Source: CAD feature listing. Evaluate the final solid. Frame: model axes, mm. Face numbers are marked on the shaded views. A direction names the side the tool comes from. Round coordinates to 2 decimals unless told otherwise and drop trailing zeros. Order: outer loops, then holes, each group sorted by start corner. A loop starts at its lowest first (then second) coordinate and runs counter-clockwise, first axis right, second up. Notation, with made-up numbers: (56, 32.25) - (100, 32.25) arc R12 ccw to (100, 37.25) - close; hole circle Ø11 at (60, -22.75). An arc over 180 degrees is marked (long way). Use one line per item in the form item = value. Start each with the question number.
Q1. Cut plane B-B, the plane y = 32. Return the cut outline in (x, z).
Q2. Ray query, line 1 (X direction, y = 16, z = 96.5); line 2 (Y direction, x = -37, z = 23); line 3 (Z direction, x = -62, y = 70). Return the intervals inside material, ascending. Write a range as [from, to].
Q3. Set-up query: the marked faces 1 and 2. Return all of +Z, -Z, +X, -X, +Y, -Y with unobstructed straight access to the full face (end or side cutting, diameter ignored); none if empty.
Q4. Cut plane C-C, the plane z = 8.5. Return the cut outline in (x, y), and give its area (3 significant figures).
Q5. Cut plane D-D, the plane x = -61.5. Return the cut outline in (y, z).
Q6. Draft query along Y for the marked faces 3, 4 and 5. Return one class per face: released by +Y, released by -Y, zero draft, split by the parting line, or undercut.
Q7. Cut plane A-A, the plane x = -28.5. Return the cut outline in (y, z), and give its area (3 significant figures).
Q8. Pin query (flat end, axial travel): pin 1 Ø0.8 at (y, z) = (0.5, 63.5) entering from -X; pin 2 Ø3 at (x, z) = (-52, 51.5) entering from -Y; pin 3 Ø1.5 at (x, y) = (-27.5, 50) entering from +Z. Return the tip coordinate at first contact, or that it passes through.
from build123d import *

# Parameters (mm, degrees)
F0_W     = 83.5
F0_H     = 82.5
F1_DEPTH = 116
F3_DEPTH = 25
F4_R     = 3
F5_DEPTH = 2
F6_R     = 4.99999


# Not quite as in the source:
# - a fillet or chamfer is up to 0.001 mm smaller than in the source, because OpenCascade refuses the exact size


with BuildPart() as f1:
    # F0 (on Top) → F1 (new body)
    with BuildSketch(Plane.XY):
        with Locations((-41.75, 41.25)):
            Rectangle(F0_W, F0_H)
        Polygon((-2, 1.5), (-43.8047535717, 1.5), (-81.5, 1.5), (-81.5, 41.25), (-81.5, 80.5), (-41.75, 80.5), (-2, 80.5), (-2, 41.25), align=None, mode=Mode.SUBTRACT)
    extrude(amount=F1_DEPTH)

    # F2 (on Front) → F3 (cut)
    with BuildSketch(Plane.XZ):
        Polygon((-5, 111), (-78.5, 111), (-78.5, 20), (-41.75, 20), (-34.1152064502, 32.9003408551), (-5, 32.9003408551), align=None)
    extrude(amount=-F3_DEPTH, mode=Mode.SUBTRACT)

    # F4
    f4_edges = [f1.edges().sort_by_distance(p)[0] for p in [
        (-34.115206, 0.75, 32.900341),
    ]]
    fillet(f4_edges, radius=F4_R)

    # F0 (on Top) → F5 (join)
    with BuildSketch(Plane.XY):
        Polygon((-81.5, 1.5), (-43.8047535717, 1.5), (-2, 1.5), (-2, 41.25), (-2, 80.5), (-41.75, 80.5), (-81.5, 80.5), (-81.5, 41.25), align=None)
    extrude(amount=F5_DEPTH)

    # F6 (radius 5 in the source; OpenCascade refuses exactly that, so slightly less here)
    f6_edges = [f1.edges().sort_by_distance(p)[0] for p in [
        (-83.5, 0, 58),
        (0, 0, 58),
        (0, 82.5, 58),
        (-83.5, 82.5, 58),
    ]]
    fillet(f6_edges, radius=F6_R)


solid = f1.part
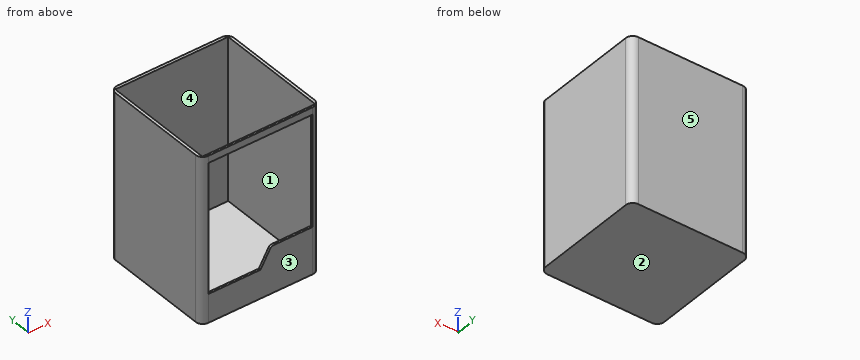
Completed:
q1.outline = (-83.5, 0) - (0, 0) - (0, 116) - (-2, 116) - (-2, 2) - (-81.5, 2) - (-81.5, 116) - (-83.5, 116) - close
q2.line_1 = [-83.5, -81.5], [-2, 0]
q2.line_2 = [0, 1.5], [80.5, 82.5]
q2.line_3 = [0, 2]
q3.face_1 = +Z
q3.face_2 = -Z, +X, -X, +Y, -Y
q4.outline = (-83.5, 5) arc R5 ccw to (-78.5, 0) - (-5, 0) arc R5 ccw to (0, 5) - (0, 77.5) arc R5 ccw to (-5, 82.5) - (-78.5, 82.5) arc R5 ccw to (-83.5, 77.5) - close; hole (-81.5, 1.5) - (-2, 1.5) - (-2, 80.5) - (-81.5, 80.5) - close
q4.area = 587 mm2
q5.outline = (0, 0) - (82.5, 0) - (82.5, 116) - (80.5, 116) - (80.5, 2) - (1.5, 2) - (1.5, 20) - (0, 20) - close; (0, 111) - (1.5, 111) - (1.5, 116) - (0, 116) - close
q6.face_3 = released by -Y
q6.face_4 = undercut
q6.face_5 = released by +Y
q7.outline = (0, 0) - (82.5, 0) - (82.5, 116) - (80.5, 116) - (80.5, 2) - (1.5, 2) - (1.5, 32.9) - (0, 32.9) - close; (0, 111) - (1.5, 111) - (1.5, 116) - (0, 116) - close
q7.area = 447 mm2
q8.pin_1 = -81.36
q8.pin_2 = 80.5
q8.pin_3 = 2
